Model file for the job. Use its own axes, mm. A direction names the side the tool comes from. Give positions to 0.01 mm unless a question says otherwise; leave off trailing zeros. Loops run counter-clockwise (first coordinate to the right, second up) from the corner with the lowest first, then second, coordinate; pieces in that order, holes last. Notation, with made-up numbers: M 36,-25 L 56,-25 A25 cw 56,-4 Z; hole C 59,2 d6. An arc over 180 degrees is marked long. Answer in a Markdown table with one row per item.
```python
from build123d import *

# Parameters (mm, degrees)
SKETCH001_R     = 6
POCKET_DEPTH    = 8.820854
CHAMFER_SIZE    = 0.2
CHAMFER001_SIZE = 1


with BuildPart() as pocket:
    # Sketch003 → Revolution001 (revolve)
    with BuildSketch(Plane.XZ):
        Polygon((0, 1.180146), (5, 3), (5, 10), (0, 10), align=None)
    revolve(axis=Axis((0, 0, 0), (0, 0, 1)))

    # Sketch001 (on Face3 of Revolution001) → Pocket (cut, through all)
    with BuildSketch(Plane(origin=(0, 0, 10), x_dir=(-1, 0, 0), z_dir=(0, 0, 1))):
        Circle(SKETCH001_R)
        Polygon((-1.443376, 2.5), (1.443376, 2.5), (2.886751, 0), (1.443376, -2.5), (-1.443376, -2.5), (-2.886751, 0), align=None, mode=Mode.SUBTRACT)
    extrude(amount=-POCKET_DEPTH, mode=Mode.SUBTRACT)


with BuildPart() as chamfer001:
    # Sketch → Revolution (revolve)
    with BuildSketch(Plane.XZ):
        Polygon((2.88675, 6), (5, 6), (5, 0), (3, 0), (3, -18), (0, -18), (0, 3.113247), align=None)
    revolve(axis=Axis((0, 0, 0), (0, 0, 1)))

    # Cut: cut Pocket
    add(pocket.part, mode=Mode.SUBTRACT)

    # Chamfer
    chamfer_edges = [chamfer001.edges().sort_by_distance(p)[0] for p in [
        (-5, 0, 6),
        (-5, 0, 0),
    ]]
    chamfer(chamfer_edges, length=CHAMFER_SIZE)

    # Chamfer001
    chamfer001_edges = [chamfer001.edges().sort_by_distance(p)[0] for p in [
        (-3, 0, -18),
    ]]
    chamfer(chamfer001_edges, length=CHAMFER001_SIZE)


solid = chamfer001.part
```
(1) Wall check: L1, parallel to Y at x = 0, z = -14.75; L2, parallel to X at y = 1.5, z = 4; L3, parallel to Z at x = 3, y = -1. Give the ranges that are in metal, low to high.
Established:
| item | result |
|---|---|
| L1 | y = -3 to 3 |
| L2 | x = -4.77 to -2.02, 2.02 to 4.77 |
| L3 | z = 0 to 6 |
(2) Which spindle directions (+Z, -Z, +X, -X, +Y, -Y) get a long thin tool onto all of the face, cutting with end or side? Do faces 4 (the conical face through (2.345, 1.331, 5.809)), 5 (the flat face through (0, 0, -18)), 6 (the cylindrical face through (-3, 0, -9)). Say none if no direction does.
Established:
| item | result |
|---|---|
| face 4 | +Z |
| face 5 | -Z, +X, -X, +Y, -Y |
| face 6 | -Z |
(3) Flat gauge pins, fed straight in: P1, Ø4, axis at y = 2.5, z = -0.5, coming from the +X side; P2, Ø1, axis at x = 0, z = -15, coming from the -Y side; P3, Ø4, axis at y = 1.5, z = -8.5, coming from the +X side. Where does each tip first touch, or does it go through?
Established:
| item | result |
|---|---|
| P1 | stops at x = 4.96 |
| P2 | stops at y = -3 |
| P3 | stops at x = 3 |
(4) Mould opens along X. For faces 1 (the flat face through (2.175, -1.233, 4.072)), 2 (the cylindrical face through (-1.08, -4.88, 2.96)), 3 (the flat face through (1, -3, 0)) say: pulls with the +X half, pulls with the -X half, needs draft (parallel to the pull), parting line crosses it, or undercut.
Established:
| item | result |
|---|---|
| face 1 | undercut |
| face 2 | parting line crosses it |
| face 3 | needs draft |
(5) Saw through at A-A, the plane z = -2.5. Give the cut face in (x, y).
Established:
| item | result |
|---|---|
| outline | C 0,0 d6 |
